from build123d import *

# Parameters (mm, degrees)
SKETCH1_W           = 38.1
SKETCH1_H           = 25.4
BOSS_EXTRUDE1_DEPTH = 25.4
SKETCH2_W           = 32.004
SKETCH2_H           = 25.4
CUT_EXTRUDE1_DEPTH  = 22.86
SKETCH3_R           = 3.302
CUT_EXTRUDE2_DEPTH  = 48.519048812
FILLET1_R           = 7.62
SKETCH4_W           = 38.1
SKETCH4_H           = 25.4
BOSS_EXTRUDE2_DEPTH = 25.4
FILLET2_R           = 7.62


with BuildPart() as part:
    # Sketch1 → Boss-Extrude1 (new body)
    with BuildSketch(Plane(origin=(0, 0, 0), x_dir=(1, 0, 0), z_dir=(0, 1, 0))):
        Rectangle(SKETCH1_W, SKETCH1_H)
    extrude(amount=BOSS_EXTRUDE1_DEPTH)

    # Sketch2 → Cut-Extrude1 (cut)
    with BuildSketch(Plane(origin=(0, 25.4, 0), x_dir=(1, 0, 0), z_dir=(0, 1, 0))):
        Rectangle(SKETCH2_W, SKETCH2_H)
    extrude(amount=-CUT_EXTRUDE1_DEPTH, mode=Mode.SUBTRACT)

    # Sketch3 → Cut-Extrude2 (cut, through all)
    with BuildSketch(Plane.ZY.offset(19.05)):
        with Locations((0, 15.24)):
            Circle(SKETCH3_R)
    extrude(amount=-CUT_EXTRUDE2_DEPTH, mode=Mode.SUBTRACT)

    # Fillet1
    fillet1_edges = [part.edges().sort_by_distance(p)[0] for p in [
        (-17.526, 25.4, -12.7),
        (17.526, 25.4, 12.7),
        (-17.526, 25.4, 12.7),
        (17.526, 25.4, -12.7),
    ]]
    fillet(fillet1_edges, radius=FILLET1_R)

    # Sketch4 → Boss-Extrude2 (add)
    with BuildSketch(Plane.XZ):
        Rectangle(SKETCH4_W, SKETCH4_H)
    extrude(amount=BOSS_EXTRUDE2_DEPTH)

    # Fillet2
    fillet2_edges = [part.edges().sort_by_distance(p)[0] for p in [
        (-19.05, -25.4, 0),
        (0, -25.4, -12.7),
        (19.05, -25.4, 0),
        (0, -25.4, 12.7),
    ]]
    fillet(fillet2_edges, radius=FILLET2_R)


solid = part.part
Source: CAD feature listing. Evaluate the final solid. Frame: model axes, mm. A direction names the side the tool comes from. Give positions to 0.01 mm unless a question says otherwise; leave off trailing zeros. Order: outer loops, then holes, each group sorted by start corner. A loop starts at its lowest first (then second) coordinate and runs counter-clockwise, first axis right, second up. Notation, with made-up numbers: (36, -4) -> (40, -4) arc R4 cw to (40, 0) -> close; hole circle Ø5 at (-11, 46.25). An arc over 180 degrees is marked (long way). Use a Markdown table: item, result.
1) Section query C-C, the plane y = 9.5. Return the cut outline in (x, z).
Answer list:
| item | result |
|---|---|
| outline | (-19.05, -12.7) -> (-16, -12.7) -> (-16, 12.7) -> (-19.05, 12.7) -> close; (16, -12.7) -> (19.05, -12.7) -> (19.05, 12.7) -> (16, 12.7) -> close |
2) Section query D-D, the plane x = 7.5. Return the cut outline in (y, z).
Answer list:
| item | result |
|---|---|
| outline | (-25.4, -5.08) arc R7.62 ccw to (-17.78, -12.7) -> (2.54, -12.7) -> (2.54, 12.7) -> (-17.78, 12.7) arc R7.62 ccw to (-25.4, 5.08) -> close |
3) Section query B-B, the plane z = 0. Return the cut outline in (x, y), then the cut area to 3 significant figures.
Answer list:
| item | result |
|---|---|
| outline | (-19.05, -17.78) arc R7.62 ccw to (-11.43, -25.4) -> (11.43, -25.4) arc R7.62 ccw to (19.05, -17.78) -> (19.05, 11.94) -> (16, 11.94) -> (16, 2.54) -> (-16, 2.54) -> (-16, 11.94) -> (-19.05, 11.94) -> close; (-19.05, 18.54) -> (-16, 18.54) -> (-16, 25.4) -> (-19.05, 25.4) -> close; (16, 18.54) -> (19.05, 18.54) -> (19.05, 25.4) -> (16, 25.4) -> close |
| area | 1,140 mm² |
4) Ray query, line 1 along X through (y, z) = (17.5, -9.75); line 2 along Z through (x, y) = (-17, 15); line 3 along Y through (x, z) = (-16.7, 0). Return the intervals inside material, ascending. Write a range as [from, to].
Answer list:
| item | result |
|---|---|
| line 1 | [-19.05, -16], [16, 19.05] |
| line 2 | [-12.7, -3.29], [3.29, 12.7] |
| line 3 | [-23.28, 11.94], [18.54, 25.4] |
5) Reachability of faces 1 (the flat face through (16.002, 11.6, 0.2)), 2 (the flat face through (0, -4, -12.7)) from +Z, -Z, +X, -X, +Y, -Y: full face, straight path, thin tool, end or side. Return the list, or none.
Answer list:
| item | result |
|---|---|
| face 1 | +Z, -Z, +Y |
| face 2 | -Z, +X, -X, +Y, -Y |
6) Mould query, pull axis Z, two halves, no side actions, for faces 3 (the cylindrical face through (17.547, 23.109, -10.527)), 4 (the flat face through (18, 25.4, 0)), 5 (the cylindrical face through (-17.547, 12.017, -0.716)), 6 (the cylindrical face through (17.505, 12.017, -0.716)). Classes: +Z half, -Z half, draft (parallel to the pull), parting line (faces both ways), or undercut.
Answer list:
| item | result |
|---|---|
| face 3 | -Z half |
| face 4 | draft |
| face 5 | undercut |
| face 6 | undercut |
7) Section query A-A, the plane y = 15.24. Return the cut outline in (x, z), then the cut area to 3 significant figures.
Answer list:
| item | result |
|---|---|
| outline | (-19.05, -12.7) -> (-16, -12.7) -> (-16, -3.3) -> (-19.05, -3.3) -> close; (-19.05, 3.3) -> (-16, 3.3) -> (-16, 12.7) -> (-19.05, 12.7) -> close; (16, -12.7) -> (19.05, -12.7) -> (19.05, -3.3) -> (16, -3.3) -> close; (16, 3.3) -> (19.05, 3.3) -> (19.05, 12.7) -> (16, 12.7) -> close |
| area | 115 mm² |
8) Contact query for flat-ended pins moving along their axis: P1, Ø7.5, axis at x = 6, z = 5.5, coming from the +Y side; P2, Ø1.5, axis at x = 11, z = 9.5, coming from the -Y side. Output: stop coordinate, or through.
Answer list:
| item | result |
|---|---|
| P1 | y = 2.54 |
| P2 | y = -24.46 |
